Geometry: final body of the model. Coordinates: model frame, mm. Face numbers are marked on the shaded views. A direction names the side the tool comes from. Give positions to 0.01 mm unless a question says otherwise; leave off trailing zeros. Order: outer loops, then holes, each group sorted by start corner. A loop starts at its lowest first (then second) coordinate and runs counter-clockwise, first axis right, second up. Notation, with made-up numbers: (63.5, 63.5) - (111.5, 63.5) arc R28 ccw to (111.5, 86.5) - close; hole circle Ø3 at (70, 8.25). An arc over 180 degrees is marked (long way). One line per item, written item: value.
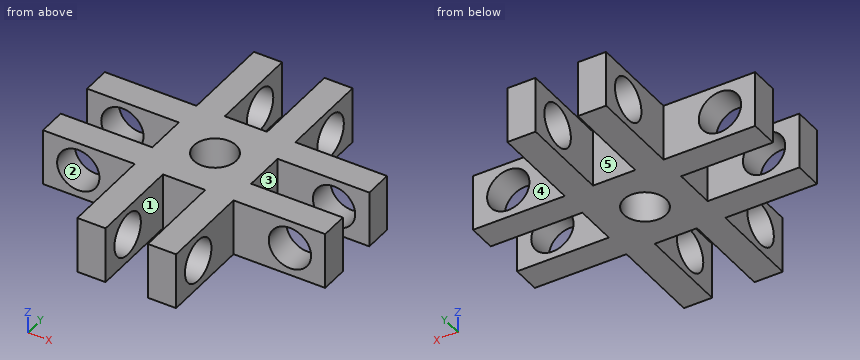
Autodesk Inventor part; units mm, degrees
ref_plane "YZ Plane" through (0, 0, 0) normal (1, 0, 0) x (0, 1, 0)
ref_plane "XZ Plane" through (0, 0, 0) normal (0, 1, 0) x (-1, 0, 0)
ref_plane "XY Plane" through (0, 0, 0) normal (0, 0, 1) x (1, 0, 0)
sketch "Sketch1" plane through (0, 0, 0) normal (0, 0, 1) x (1, 0, 0)
  line L0 (0, 0) -> (20, 0)
  line L1 (20, 0) -> (20, 20)
  line L2 (20, 20) -> (0, 20)
  line L3 (0, 20) -> (0, 0)
  line L4 (8.4977, 20) -> (6.4977, 20)
  line L5 (6.4977, 0) -> (8.4977, 0)
  line L6 (0, 3.9) -> (0, 5.9)
  line L7 (20, 8.9) -> (20, 10.9)
  line L8 (0, 10.9) -> (0, 8.9)
  line L9 (10, 0) -> (10, 10)
  circle A0 centre (10, 10) radius 1.5
  line L10 (0, 11.5) -> (20, 11.5)
  line L11 (20, 11.5) -> (20, 13.5)
  line L12 (20, 13.5) -> (0, 13.5)
  line L13 (0, 13.5) -> (0, 11.5)
  line L14 (6.5, 20) -> (6.5, 0)
  line L15 (8.5, 0) -> (8.5, 20)
  line L16 (0, 6.5) -> (20, 6.5)
  line L17 (20, 8.5) -> (0, 8.5)
  line L18 (13.5, 0) -> (13.5, 20)
  line L19 (11.5, 20) -> (11.5, 0)
  point P0 (6.5, 11.5)
  point P1 (6.5, 8.5)
  point P2 (6.5, 6.5)
  point P3 (6.5, 0)
  point P4 (8.5, 6.5)
  point P5 (10, 6.5)
  point P6 (13.5, 6.5)
  point P7 (13.5, 8.5)
  point P8 (13.5, 11.5)
  point P9 (13.5, 13.5)
  point P10 (11.5, 13.5)
  point P11 (8.5, 13.5)
  point P12 (6.5, 13.5)
  point P13 (0, 13.5)
  point P14 (11.5, 6.5)
  dimension "d0" = 20
  dimension "d1" = 20
  dimension "d7" = 2
  dimension "d10" = 2
  dimension "d19" = 10
  dimension "d20" = 3
  dimension "d21" = 20
  dimension "d22" = 2
  dimension "d25" = 360
extrude "Extrusion1" add sketch "Sketch1" along normal blind 4 contours L14 L16 L15 L0 | L16 L3 L17 L14 | L14 L17 L15 L16 | L14 L10 L15 L17 | L15 L17 L9 L16 | L14 L12 L15 L10 | L10 L3 L12 L14 | L15 A0 L17 | L9 L17 L19 L16 | L19 L16 L18 L0 | L15 L12 L19 L10 | L10 A0 L15 | L14 L2 L15 L12 | A0 L19 L17 | L19 L17 L18 L16 | L10 L19 A0 | L19 L10 L18 L17 | L18 L17 L1 L16 | L19 L12 L18 L10 | L19 L2 L18 L12 | L18 L12 L1 L10
sketch "Sketch3" plane through (13.5, 6.5, 0) normal (0, -1, 0) x (1, 0, 0)
  line L0 (0, 0) -> (0, 4)
  line L1 (0, 0) -> (4, 0)
  line L2 (0, 0) -> (6.5, 0)
  line L3 (4, 0) -> (4, 2)
  circle A0 centre (4, 2) radius 1.5
  point P0 (-13.5, 0)
  dimension "d27" = 4
  dimension "d28" = 2
  dimension "d29" = 3
extrude "Extrusion3" cut sketch "Sketch3" against normal blind 10
pattern_circular "Circular Pattern2" count 4 over 360 about axis through (10, 10, 0) along (0, 0, 1) of "Extrusion3"
properties part number "Center Connector"
1) Section A-A, the plane y = 17.5. Return loops of the section in (x, z), then the cut area to 3 significant figures.
Answers below:
outline: (6.5, 0) - (8.5, 0) - (8.5, 0.5) - (6.5, 0.5) - close; (6.5, 3.5) - (8.5, 3.5) - (8.5, 4) - (6.5, 4) - close; (11.5, 0) - (13.5, 0) - (13.5, 0.5) - (11.5, 0.5) - close; (11.5, 3.5) - (13.5, 3.5) - (13.5, 4) - (11.5, 4) - close
area: 4.00 mm^2
2) Set-up query: the marked faces 3, 4 and 5. Return all of +Z, -Z, +X, -X, +Y, -Y with unobstructed straight access to the full face (end or side cutting, diameter ignored); none if empty.
Answers below:
face 3: +Z, -Z, +X
face 4: +Z, -Z, +X, +Y
face 5: +Z, -Z, +Y
3) Section B-B, the plane x = 10. Return loops of the section in (y, z), then the cut area to 3 significant figures.
Answers below:
outline: (6.5, 0) - (8.5, 0) - (8.5, 4) - (6.5, 4) - close; (11.5, 0) - (13.5, 0) - (13.5, 4) - (11.5, 4) - close
area: 16.0 mm^2
4) First-contact query: pin 1 (2 mm diameter, centred on x = 16, z = 2.5, fed in from +Y); pin 2 (1.2 mm diameter, centred on y = 1.5, z = 1.5, fed in from +X); pin 3 (1.2 mm diameter, centred on x = 2.5, z = 2, fed in from +Y); pin 4 (2 mm diameter, centred on y = 2, z = 3, fed in from -X). Flat tips, straight axial feed; report the tip coordinate or a pass-through.
Answers below:
pin 1: y = 13.5
pin 2: x = 13.5
pin 3: through
pin 4: x = 6.5
5) Mould query, pull axis Z, two halves, no side actions, for the marked faces 1 and 2. Classes: released by +Z, released by -Z, zero draft, split by the parting line, or undercut.
Answers below:
face 1: zero draft
face 2: undercut
6) Material intervals for line 1 along Y through (x, z) = (12.95, 2); line 2 along X through (y, z) = (14.75, 1.7), sorted ascending.
Answers below:
line 1: 0 to 1, 4 to 16, 19 to 20
line 2: 6.5 to 8.5, 11.5 to 13.5
